```python
from build123d import *

# Parameters (mm, degrees)
EXTRUDE_2_DEPTH     = 7
EXTRUDE_START       = -2
EXTRUDE_3_DEPTH     = 2
EXTRUDE_4_DEPTH     = 1
SKETCH_11_R         = 1.5
SKETCH_11_R_2       = 1
CUT_EXTRUDE_2_DEPTH = 2
CUT_EXTRUDE_3_DEPTH = 1


with BuildPart() as part:
    # ｽｹｯﾁ7 → ﾎﾞｽ - 押し出し2 (new body)
    with BuildSketch(Plane(origin=(0, 0, 0), x_dir=(1, 0, 0), z_dir=(0, 1, 0))):
        with BuildLine():
            Line((22, 25.2), (0, 25.2))
            Line((0, 25.2), (0, 27))
            Line((0, 27), (22, 27))
            ThreePointArc((22, 27), (25.535533906, 25.535533906), (27, 22))
            Line((27, 22), (27, 0))
            Line((27, 0), (25.2, 0))
            Line((25.2, 0), (25.2, 22))
            ThreePointArc((25.2, 22), (24.2627417, 24.2627417), (22, 25.2))
        make_face()
    extrude(amount=EXTRUDE_2_DEPTH)

    # ｽｹｯﾁ8 → ﾎﾞｽ - 押し出し3 (add)
    with BuildSketch(Plane(origin=(0, 7, 0), x_dir=(1, 0, 0), z_dir=(0, 1, 0)).offset(EXTRUDE_START)):
        with BuildLine():
            Line((15.2, 21.2), (15.2, 25.2))
            Line((15.2, 25.2), (22, 25.2))
            ThreePointArc((22, 25.2), (24.2627417, 24.2627417), (25.2, 22))
            Line((25.2, 22), (25.2, 18.2))
            Line((25.2, 18.2), (18.2, 18.2))
            ThreePointArc((18.2, 18.2), (16.078679656, 19.078679656), (15.2, 21.2))
        make_face()
    extrude(amount=EXTRUDE_3_DEPTH)

    # ｽｹｯﾁ10 → ﾎﾞｽ - 押し出し4 (add)
    with BuildSketch(Plane(origin=(0, 7, 0), x_dir=(1, 0, 0), z_dir=(0, 1, 0))):
        with BuildLine():
            Line((25, 23.2), (25, 18.2))
            Line((25, 18.2), (25.5, 18.2))
            Line((25.5, 18.2), (25.5, 22))
            ThreePointArc((25.5, 22), (24.474873734, 24.474873734), (22, 25.5))
            Line((22, 25.5), (15.2, 25.5))
            Line((15.2, 25.5), (15.2, 25))
            Line((15.2, 25), (23.2, 25))
            Line((23.2, 25), (25, 23.2))
        make_face()
    extrude(amount=EXTRUDE_4_DEPTH)

    # ｽｹｯﾁ11 → ｶｯﾄ - 押し出し2 (cut)
    with BuildSketch(Plane(origin=(0, 7, 0), x_dir=(1, 0, 0), z_dir=(0, 1, 0))):
        with Locations(Location((22, 22, 0), (0, 0, 270))):
            Circle(SKETCH_11_R)
        with Locations(Location((18, 22, 0), (0, 0, 270))):
            Circle(SKETCH_11_R_2)
    extrude(amount=-CUT_EXTRUDE_2_DEPTH, mode=Mode.SUBTRACT)

    # ｽｹｯﾁ12 → ｶｯﾄ - 押し出し3 (cut)
    with BuildSketch(Plane(origin=(0, 0, 0), x_dir=(-1, 0, 0), z_dir=(0, -1, 0))):
        with BuildLine():
            Line((-22, 25), (-15.2, 25))
            Line((-15.2, 25), (-15.2, 25.5))
            Line((-15.2, 25.5), (-22, 25.5))
            ThreePointArc((-22, 25.5), (-24.474873734, 24.474873734), (-25.5, 22))
            Line((-25.5, 22), (-25.5, 18.2))
            Line((-25.5, 18.2), (-25, 18.2))
            Line((-25, 18.2), (-25, 22))
            ThreePointArc((-25, 22), (-24.121320344, 24.121320344), (-22, 25))
        make_face()
    extrude(amount=-CUT_EXTRUDE_3_DEPTH, mode=Mode.SUBTRACT)

    # ﾐﾗｰ1: part across plane


with BuildPart() as part_1:
    add(part.part)
    add(part.part.mirror(Plane(origin=(0, 0, 0), x_dir=(0, 0, 1), z_dir=(1, 0, 0))))

    # ﾐﾗｰ2: part across plane


with BuildPart() as part_2:
    add(part_1.part)
    add(part_1.part.mirror(Plane.XY))


solid = part_2.part
```
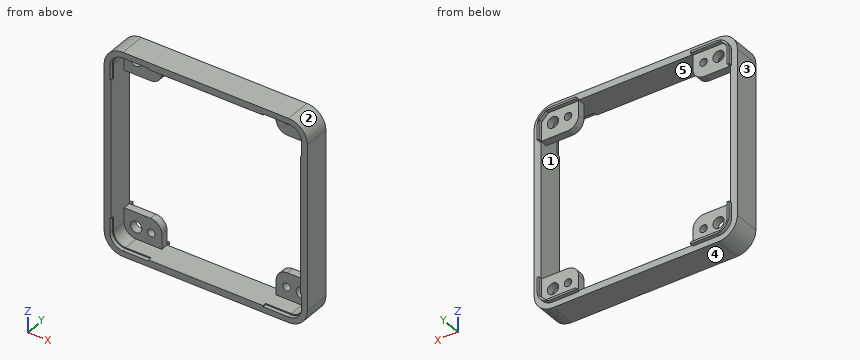
CAD build for the part. Positions are in the model's coordinates, mm. Face numbers are marked on the shaded views. A direction names the side the tool comes from. Round coordinates to 2 decimals unless told otherwise and drop trailing zeros. Order: outer loops, then holes, each group sorted by start corner. A loop starts at its lowest first (then second) coordinate and runs counter-clockwise, first axis right, second up.
Q1. Which spindle directions (+Z, -Z, +X, -X, +Y, -Y) get a long thin tool onto all of the face, cutting with end or side? Do the marked faces 4 and 5. Say none if no direction does.
Q2. Slice it at B-B (z = 5.5). Write the cut outline in (x, y).
Q3. Drop flat-ended pins along their axis: pin 1 (0.8 mm diameter, centred on x = -17.5, y = 7.5, fed in from +Z); pin 2 (1.5 mm diameter, centred on y = 6.5, z = -23.5, fed in from -X); pin 3 (0.9 mm diameter, centred on x = 23.5, y = 7, fed in from +Z). Give the stop position or say it passes through.
Q4. Two-plate mould, pull along Z, no slides. Class the marked faces 1, 2 and 3: pulls with the +Z half, pulls with the -Z half, needs draft (parallel to the pull), parting line crosses it, or undercut.
Q5. Slice it at A-A (x = -1.5). Write the cut outline in (y, z), and give its area (3 significant figures).
Q6. Wall check: L1, parallel to X at y = 5.55, z = 22; L2, parallel to Z at x = -18, y = 6.2; L3, parallel to Z at x = -22, y = 5.75. Give the ranges that are in metal, low to high.
Q7. Slice it at C-C (y = 3.75). Write the cut outline in (x, z), and give its area (3 significant figures).
Results below:
1. face 4: -Z, +X, -X, +Y, -Y
1. face 5: -Y
2. outline: (-27, 0) - (-25.2, 0) - (-25.2, 7) - (-27, 7) - close; (25.2, 0) - (27, 0) - (27, 7) - (25.2, 7) - close
3. pin 1: stops at z = 25.5
3. pin 2: stops at x = -26.94
3. pin 3: stops at z = 26.89
4. face 1: undercut
4. face 2: pulls with the +Z half
4. face 3: needs draft
5. outline: (0, -27) - (7, -27) - (7, -25.2) - (0, -25.2) - close; (0, 25.2) - (7, 25.2) - (7, 27) - (0, 27) - close
5. area: 25.2 mm2
6. L1: x = -27 to -23.5, -20.5 to -19, -17 to -15.2, 15.2 to 17, 19 to 20.5, 23.5 to 27
6. L2: z = -27 to -23, -21 to -18.21, 18.21 to 21, 23 to 27
6. L3: z = -27 to -23.5, -20.5 to -18.2, 18.2 to 20.5, 23.5 to 27
7. outline: (-27, -22) arc R5 ccw to (-22, -27) - (22, -27) arc R5 ccw to (27, -22) - (27, 22) arc R5 ccw to (22, 27) - (-22, 27) arc R5 ccw to (-27, 22) - close; hole (-25.2, -22) arc R3.2 ccw to (-22, -25.2) - (22, -25.2) arc R3.2 ccw to (25.2, -22) - (25.2, 22) arc R3.2 ccw to (22, 25.2) - (-22, 25.2) arc R3.2 ccw to (-25.2, 22) - close
7. area: 363 mm2
